Part print with two shaded views. Sizes in mm from the minimum x, y, z corner. A direction names the side the tool comes from. Coordinates: 2 decimals unless noted, no trailing zeros. Loops run counter-clockwise (first coordinate to the right, second up) from the corner with the lowest first, then second, coordinate; pieces in that order, holes last.
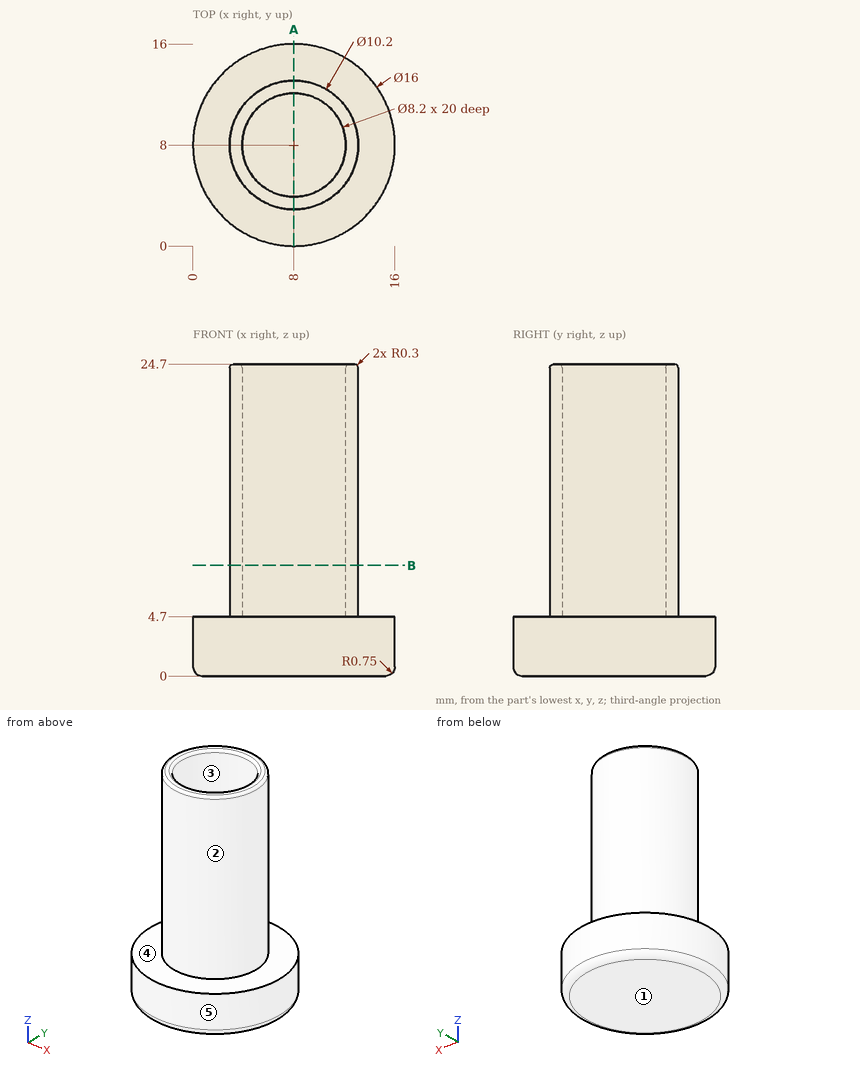
Q1. Slice it at B-B (z = 8.75). List the corners of the cut face in (x, y), and give its area (3 significant figures).
Answers:
outline: circle Ø10.2 at (8, 8); hole circle Ø8.2 at (8, 8)
area: 28.9 mm2
Q2. Slice it at A-A (x = 8). List the corners of the cut face in (y, z), and give its area (3 significant figures).
Answers:
outline: (0, 0.75) arc R0.75 ccw to (0.75, 0) - (15.25, 0) arc R0.75 ccw to (16, 0.75) - (16, 4.7) - (13.1, 4.7) - (13.1, 24.4) arc R0.3 ccw to (12.8, 24.7) - (12.4, 24.7) arc R0.3 ccw to (12.1, 24.4) - (12.1, 4.7) - (3.9, 4.7) - (3.9, 24.4) arc R0.3 ccw to (3.6, 24.7) - (3.2, 24.7) arc R0.3 ccw to (2.9, 24.4) - (2.9, 4.7) - (0, 4.7) - close
area: 115 mm2
Q3. Drill centre lines: line 1 (Y direction, x = 8, z = 19); line 2 (Z direction, x = 13.5, y = 5.75); line 3 (Y direction, x = 5.5, z = 10.25). Where is each one in solid material? Low to high.
Answers:
line 1: y = 2.9 to 3.9, 12.1 to 13.1
line 2: z = 0 to 4.7
line 3: y = 3.55 to 4.75, 11.25 to 12.45
Q4. Mould opens along Y. For the marked faces 1, 2 and 3 say: +Y half, -Y half, draft (parallel to the pull), parting line (faces both ways), or undercut.
Answers:
face 1: draft
face 2: parting line
face 3: undercut
Q5. Which spindle directions (+Z, -Z, +X, -X, +Y, -Y) get a long thin tool onto all of the face, cutting with end or side? Do the marked faces 4 and 5. Say none if no direction does.
Answers:
face 4: +Z
face 5: +Z, -Z
Q6. Flat gauge pins, fed straight in: P1, Ø6, axis at y = 9.5, z = 9.5, coming from the +X side; P2, Ø6, axis at y = 13.5, z = 20.5, coming from the -X side; P3, Ø8, axis at x = 14.5, z = 3, coming from the +Y side. Where does each tip first touch, or does it go through?
Answers:
P1: stops at x = 13.1
P2: stops at x = 3.55
P3: stops at y = 15.6
